Source: CAD feature listing. Evaluate the final solid. Frame: model axes, mm. Give positions to 0.01 mm unless a question says otherwise; leave off trailing zeros. Loops run counter-clockwise (first coordinate to the right, second up) from the corner with the lowest first, then second, coordinate; pieces in that order, holes last. Notation, with made-up numbers: M -2.75,6.25 L 56.25,6.25 A18 ccw 56.25,11.25 Z; hole C 15,32 d11. An arc over 180 degrees is marked long. Put each result on its own line as item: value. Start each with the question number.
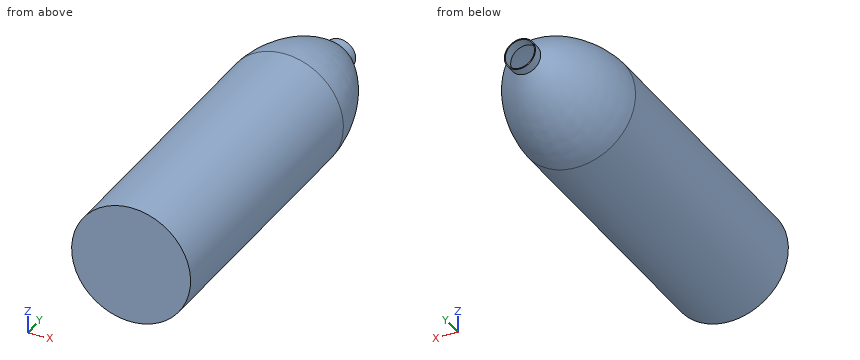
```python
from build123d import *


with BuildPart() as part:
    # Sketch8 → Revolve1 (revolve)
    with BuildSketch(Plane.XY, mode=Mode.PRIVATE) as revolve1_sk:
        with BuildLine():
            Line((0, -44.157655741), (-60, -44.157655741))
            Line((-60, -44.157655741), (-60, 255.842344259))
            ThreePointArc((-60, 255.842344259), (-46.807103103, 310.030540655), (-15, 355.842344259))
            Line((-15, 355.842344259), (-15, 365.473388744))
            Line((-15, 365.473388744), (-15, 366.473388744))
            Line((-15, 366.473388744), (-16, 366.473388744))
            Line((-16, 366.473388744), (-16, 356.258998247))
            ThreePointArc((-16, 356.258998247), (-47.810277996, 310.237725941), (-61, 255.869697429))
            Line((-61, 255.869697429), (-61, -45.157655741))
            Line((-61, -45.157655741), (0, -45.157655741))
            Line((0, -45.157655741), (0, -44.157655741))
        make_face()
    revolve(revolve1_sk.sketch.rotate(Axis((0, 434.739798995, 0), (0, -1, 0)), 270), axis=Axis((0, 434.739798995, 0), (0, -1, 0)))


solid = part.part
```
1. Section A-A, the plane y = 179.5. Output: boundary loops of the cut face in (x, z).
2. Contact query for flat-ended pins moving along their axis: pin 1 (2 mm diameter, centred on x = 13.5, y = 7, fed in from +Z); pin 2 (1.5 mm diameter, centred on x = -39, y = 52, fed in from +Z); pin 3 (1.5 mm diameter, centred on x = -12, y = 203, fed in from +Z). Output: stop coordinate, or through.
3. Ray query, line 1 (X direction, y = 60, z = 0); line 2 (X direction, y = 358, z = 0); line 3 (Y direction, x = 7, z = 13). Return the intervals inside material, ascending.
Results found:
1. outline: C 0,0 d122; hole C 0,0 d120
2. pin 1: z = 59.71
2. pin 2: z = 47.52
2. pin 3: z = 59.95
3. line 1: -61 to -60, 60 to 61
3. line 2: -16 to -15, 15 to 16
3. line 3: -45.16 to -44.16
